from build123d import *

# Parameters (mm, degrees)
F0_R     = 75
F1_DEPTH = 5
F2_R     = 4.1
F3_DEPTH = 5


with BuildPart() as f1:
    # F0 (on Top) → F1 (new body)
    with BuildSketch(Plane.XY):
        Circle(F0_R)
    extrude(amount=F1_DEPTH)

    # F2 (on face) → F3 (cut, through all)
    with BuildSketch(Plane.XY.offset(5)):
        with Locations((0, 60)):
            Circle(F2_R)
        with Locations((60, 0)):
            Circle(F2_R)
        with Locations((0, -60)):
            Circle(F2_R)
        with Locations((-60, 0)):
            Circle(F2_R)
        with BuildLine():
            ThreePointArc((74.673333, -6.992374), (75, 0), (74.673333, 6.992374))
            ThreePointArc((74.673333, 6.992374), (68, 0), (74.673333, -6.992374))
        make_face()
        with BuildLine():
            ThreePointArc((-6.992374, 74.673333), (0, 68), (6.992374, 74.673333))
            ThreePointArc((6.992374, 74.673333), (0, 75), (-6.992374, 74.673333))
        make_face()
        with BuildLine():
            ThreePointArc((-74.673333, -6.992374), (-68, 0), (-74.673333, 6.992374))
            ThreePointArc((-74.673333, 6.992374), (-75, 0), (-74.673333, -6.992374))
        make_face()
        with BuildLine():
            ThreePointArc((6.992374, -74.673333), (0, -68), (-6.992374, -74.673333))
            ThreePointArc((-6.992374, -74.673333), (0, -75), (6.992374, -74.673333))
        make_face()
    extrude(amount=-F3_DEPTH, mode=Mode.SUBTRACT)


solid = f1.part
The listing builds one solid part. Answer for the finished solid, in the listing's coordinates (mm). Round coordinates to 2 decimals unless told otherwise and drop trailing zeros. Write each loop counter-clockwise with the first axis right and the second up, starting at its lowest first coordinate (ties: lowest second). Pieces come first, ordered by that corner, then holes. Notation, with made-up numbers: M 66.5,-21 L 118.5,-21 A20 ccw 118.5,14 Z; hole C 74,20.5 d9. An arc over 180 degrees is marked long. Write each question's results on one line, items separated by ' | '. Start each with the question number.
Item 1: A cutting plane is placed at C-C on y = 0. Write down the section's boundary in (x, z), and give its area (3 significant figures).
Item 2: A cutting plane is placed at A-A on y = -60. Write down the section's boundary in (x, z), and give its area (3 significant figures).
Item 3: Straight lines are drawn through the part: L1, parallel to Y at x = -60, z = 1.35; L2, parallel to X at y = 57, z = 2; L3, parallel to Y at x = 45.5, z = 3.6. For each, find the intervals that lie inside material, in ascending order. Write a range as [from, to].
Item 4: Flat-ended cylindrical pins translate along their axes: pin 1 Ø6.5 at (x, y) = (-60, 0) entering from +Z; pin 2 Ø2 at (y, z) = (-54, 4) entering from +X; pin 3 Ø3 at (x, z) = (34, 4.5) entering from +Y; pin 4 Ø1 at (x, z) = (26, 1.5) entering from -Y. Find the tip coordinate at first contact, or state that the pin passes through.
Item 5: A cutting plane is placed at D-D on z = 3.5. Write down the section's boundary in (x, y), and give its area (3 significant figures).
Item 6: For a pull along X with two mould halves and no side action, classify faces 1 (the face through (-0.534, -55.935, 2.535)), 2 (the face through (52.52, -53.54, 2.46)), 3 (the face through (-1, 1, 5)), 4 (the face through (-53.54, -52.52, 2.46)) as pulls with the +X half, pulls with the -X half, needs draft (parallel to the pull), parting line crosses it, or undercut.
Check sheet entries:
1) outline: M -68,0 L -64.1,0 L -64.1,5 L -68,5 Z; M -55.9,0 L 55.9,0 L 55.9,5 L -55.9,5 Z; M 64.1,0 L 68,0 L 68,5 L 64.1,5 Z | area: 598 mm²
2) outline: M -45,0 L -4.1,0 L -4.1,5 L -45,5 Z; M 4.1,0 L 45,0 L 45,5 L 4.1,5 Z | area: 409 mm²
3) L1: [-45, -4.1], [4.1, 45] | L2: [-48.74, -2.79], [2.79, 48.74] | L3: [-59.62, 59.62]
4) pin 1: through | pin 2: x = 53.07 | pin 3: y = 67.59 | pin 4: y = -70.53
5) outline: M -74.67,-6.99 A75 ccw -6.99,-74.67 A7 cw 6.99,-74.67 A75 ccw 74.67,-6.99 A7 cw 74.67,6.99 A75 ccw 6.99,74.67 A7 cw -6.99,74.67 A75 ccw -74.67,6.99 A7 cw Z; hole C -60,0 d8.2; hole C 0,-60 d8.2; hole C 0,60 d8.2; hole C 60,0 d8.2 | area: 17,200 mm²
6) face 1: undercut | face 2: pulls with the +X half | face 3: needs draft | face 4: pulls with the -X half
